Here's how the part is built. I have some questions about the finished solid (model axes, mm). A direction names the side the tool comes from. Give positions to 0.01 mm unless a question says otherwise; leave off trailing zeros. Loops run counter-clockwise (first coordinate to the right, second up) from the corner with the lowest first, then second, coordinate; pieces in that order, holes last. Notation, with made-up numbers: (52, 67) - (109, 67) arc R8 ccw to (109, 74) - close; hole circle Ø1 at (37.25, 82). An arc over 180 degrees is marked (long way). One line per item, written item: value. Start each with the question number.
```python
from build123d import *

# Parameters (mm, degrees)
SKETCH1_R           = 13.7
BOSS_EXTRUDE1_DEPTH = 38
SKETCH2_R           = 18.5
BOSS_EXTRUDE2_DEPTH = 22
SKETCH3_R           = 6
BOSS_EXTRUDE3_DEPTH = 6.8
SKETCH4_R           = 3
BOSS_EXTRUDE4_DEPTH = 30
SKETCH5_R           = 1.5
CUT_EXTRUDE1_DEPTH  = 5


with BuildPart() as part:
    # Sketch1 → Boss-Extrude1 (new body)
    with BuildSketch(Plane.XY):
        Circle(SKETCH1_R)
    extrude(amount=BOSS_EXTRUDE1_DEPTH)

    # Sketch2 → Boss-Extrude2 (add)
    with BuildSketch(Plane.XY.offset(38)):
        Circle(SKETCH2_R)
    extrude(amount=BOSS_EXTRUDE2_DEPTH)

    # Sketch3 → Boss-Extrude3 (add)
    with BuildSketch(Plane.XY.offset(60)):
        with Locations((0, 7)):
            Circle(SKETCH3_R)
    extrude(amount=BOSS_EXTRUDE3_DEPTH)

    # Sketch4 → Boss-Extrude4 (add)
    with BuildSketch(Plane.XY.offset(66.8)):
        with Locations((0, 7)):
            Circle(SKETCH4_R)
    extrude(amount=BOSS_EXTRUDE4_DEPTH)

    # Sketch5 → Cut-Extrude1 (cut)
    with BuildSketch(Plane.XY.offset(60)):
        with Locations((-15.75, 0)):
            Circle(SKETCH5_R)
        with Locations((-7.875, 13.63990011)):
            Circle(SKETCH5_R)
        with Locations((7.875, 13.63990011)):
            Circle(SKETCH5_R)
        with Locations((15.75, 0)):
            Circle(SKETCH5_R)
        with Locations((7.875, -13.63990011)):
            Circle(SKETCH5_R)
        with Locations((-7.875, -13.63990011)):
            Circle(SKETCH5_R)
    extrude(amount=-CUT_EXTRUDE1_DEPTH, mode=Mode.SUBTRACT)


solid = part.part
```
(1) If we section it at B-B on y = 0: List the corners of the cut face in (x, z) for me, plus the area to 3 significant figures.
(2) Will these pins go through, and if not, where does the flat tip stop? pin 1 (0.9 mm diameter, centred on x = 16, y = 0, fed in from +Z); pin 2 (8 mm diameter, centred on x = -9, z = 18, fed in from -Y) (3 decimals); pin 3 (12 mm diameter, centred on y = 0.5, z = 49.5, fed in from +X); pin 4 (2.5 mm diameter, centred on x = 7.88, y = -13.64, fed in from -Z).
(3) For faces 5 (the face through (-8, -14, 55)), 6 (the face through (0, 7, 96.8)), 7 (the face through (-14, 0, 38)), which set-ups out of +Z, -Z, +X, -X, +Y, -Y let a thin tool reach every point of the face, with its end or its side?
(4) If we section it at C-C on z = 73: List the corners of the cut face in (x, y) for me, plus the area to 3 significant figures.
(5) If we section it at D-D on x = -15.75: List the corners of the cut face in (y, z) for me.
(6) If we mould it in two halves opening along X, with no side actions, what happens to faces 1 (the face through (0, 0, 0)), 2 (the face through (6.769, -12.626, 57.535)), 3 (the face through (-3, 7, 82)), 4 (the face through (-17.25, 0.07, 57.54))? For each: pulls with the +X half, pulls with the -X half, needs draft (parallel to the pull), parting line crosses it, or undercut.
(7) Please list where these lines run through material, in increasing order: probe 1 along Z at (x, y) = (6.5, -14); probe 2 along Z at (x, y) = (-7, 8); probe 3 along Y at (x, z) = (15.75, 57.5). Write a range as from..to.
(8) If we section it at A-A on x = 0: List the corners of the cut face in (y, z) for me, plus the area to 3 significant figures.
Found:
1. outline: (-18.5, 38) - (-13.7, 38) - (-13.7, 0) - (13.7, 0) - (13.7, 38) - (18.5, 38) - (18.5, 60) - (17.25, 60) - (17.25, 55) - (14.25, 55) - (14.25, 60) - (-14.25, 60) - (-14.25, 55) - (-17.25, 55) - (-17.25, 60) - (-18.5, 60) - close
1. area: 1,830 mm^2
2. pin 1: z = 55
2. pin 2: y = -12.755
2. pin 3: x = 18.5
2. pin 4: z = 38
3. face 5: +Z
3. face 6: +Z, +X, -X, +Y, -Y
3. face 7: -Z
4. outline: circle Ø6 at (0, 7)
4. area: 28.3 mm^2
5. outline: (-9.71, 38) - (9.71, 38) - (9.71, 60) - (1.5, 60) - (1.5, 55) - (-1.5, 55) - (-1.5, 60) - (-9.71, 60) - close
6. face 1: needs draft
6. face 2: undercut
6. face 3: parting line crosses it
6. face 4: undercut
7. probe 1: 38..55
7. probe 2: 0..60
7. probe 3: -9.71..-1.5, 1.5..9.71
8. outline: (-18.5, 38) - (-13.7, 38) - (-13.7, 0) - (13.7, 0) - (13.7, 38) - (18.5, 38) - (18.5, 60) - (13, 60) - (13, 66.8) - (10, 66.8) - (10, 96.8) - (4, 96.8) - (4, 66.8) - (1, 66.8) - (1, 60) - (-18.5, 60) - close
8. area: 2,120 mm^2
